Here's how the part is built. I have some questions about the finished solid (model axes, mm). Round coordinates to 2 decimals unless told otherwise and drop trailing zeros. Loops run counter-clockwise (first coordinate to the right, second up) from the corner with the lowest first, then second, coordinate; pieces in that order, holes last. Notation, with made-up numbers: M -37.5,42 L -27.5,42 A22 cw -27.5,60 Z; hole C 87.25,28.25 d11. An arc over 180 degrees is marked long. Answer as a JSON object with one key per item and string values.
Autodesk Inventor part; units mm, degrees
ref_plane "YZ Plane" through (0, 0, 0) normal (1, 0, 0) x (0, 1, 0)
ref_plane "XZ Plane" through (0, 0, 0) normal (0, 1, 0) x (-1, 0, 0)
ref_plane "XY Plane" through (0, 0, 0) normal (0, 0, 1) x (1, 0, 0)
sketch "스케치1" plane through (0, 0, 0) normal (1, 0, 0) x (0, 1, 0)
  line L0 (-6, 16.2) -> (-3, 16.2)
  line L1 (-3, 16.2) -> (0, 16.2)
  circle A0 centre (-3, 16.2) radius 1.5
  line L2 (-3, 16.2) -> (-3, 29.7)
  circle A1 centre (-3, 29.7) radius 1.5
  line L3 (-3, 16.2) -> (-3, 2.7)
  circle A2 centre (-3, 2.7) radius 1.5
  line L4 (-3, 29.7) -> (-3, 32.4)
  line L5 (-3, 32.4) -> (0, 32.4)
  line L6 (-3, 2.7) -> (-3, 0)
  line L7 (-3, 0) -> (0, 0)
  line L8 (0, 0) -> (0, 32.4)
  line L9 (-3, 32.4) -> (-6, 32.4)
  line L10 (-6, 0) -> (-3, 0)
  line L11 (-6, 0) -> (-6, 32.4)
  dimension "d0" = 3
  dimension "d1" = 3
  dimension "d2" = 3
  dimension "d3" = 13.5
  dimension "d4" = 3
  dimension "d5" = 13.5
  dimension "d6" = 3
  dimension "d7" = 2.7
  dimension "d8" = 2.7
extrude "돌출1" add sketch "스케치1" along normal blind 2.5 contours L11 L9 L4 A1 L2 A0 L0 | L0 A0 L3 A2 L6 L10 L11 | L2 A1 L4 L5 L8 L1 A0 | A0 L1 L8 L7 L6 A2 L3
chamfer "모따기1" distance 0.5 angle 45 4 edges at (0, 0, 16.2) (0, -1.5, 0) (0, -6, 16.2) (0, -4.5, 32.4)
properties part number "x 캐리지 벨트고정"
Item 1: If I drill on L1, parallel to Z at x = 0.75, y = -3; L2, parallel to Z at x = 1.8, y = -3.6; L3, parallel to Y at x = 1.3, z = 2.7, over which ranges is the centre line in solid material (lowest first)? Write a range as from..to.
Solution:
{"L1": "z = 0..1.2, 4.2..14.7, 17.7..28.2, 31.2..32.4", "L2": "z = 0..1.33, 4.07..14.83, 17.57..28.33, 31.07..32.4", "L3": "y = -6..-4.5, -1.5..0"}
Item 2: I want a section at D-D on z = 22. List the corners of the cut face in (x, y) for me, plus the area to 4 significant figures.
Solution:
{"outline": "M 0,-5.5 L 0.5,-6 L 2.5,-6 L 2.5,0 L 0.5,0 L 0,-0.5 Z", "area": "14.75 mm2"}
Item 3: We'd pull the mould along Y, two halves only. Please class faces 1 (the face through (1.232, -2.194, 28.435)), 2 (the face through (2.5, -5, 16)), 3 (the face through (1, -6, 16)): +Y half, -Y half, draft (parallel to the pull), parting line (faces both ways), or undercut.
Solution:
{"face 1": "undercut", "face 2": "draft", "face 3": "-Y half"}
Item 4: For P1, Ø2.5, axis at y = -3, z = 29.7, coming from the -X side, with a flat end and sliding along its axis, tell me the tip position at first contact or that it passes through.
Solution:
{"P1": "passes through"}
Item 5: I want a section at A-A on y = -3. List the corners of the cut face in (x, z) for me, plus the area to 4 significant figures.
Solution:
{"outline": "M 0,0.5 L 0.5,0 L 2.5,0 L 2.5,1.2 L 0,1.2 Z; M 0,4.2 L 2.5,4.2 L 2.5,14.7 L 0,14.7 Z; M 0,17.7 L 2.5,17.7 L 2.5,28.2 L 0,28.2 Z; M 0,31.2 L 2.5,31.2 L 2.5,32.4 L 0.5,32.4 L 0,31.9 Z", "area": "58.25 mm2"}
Item 6: I want a section at B-B on x = 1.6. List the corners of the cut face in (y, z) for me.
Solution:
{"outline": "M -6,0 L 0,0 L 0,32.4 L -6,32.4 Z; hole C -3,2.7 d3; hole C -3,16.2 d3; hole C -3,29.7 d3"}
Item 7: I want a section at C-C on z = 16.2. List the corners of the cut face in (x, y) for me.
Solution:
{"outline": "M 0,-5.5 L 0.5,-6 L 2.5,-6 L 2.5,-4.5 L 0,-4.5 Z; M 0,-1.5 L 2.5,-1.5 L 2.5,0 L 0.5,0 L 0,-0.5 Z"}
